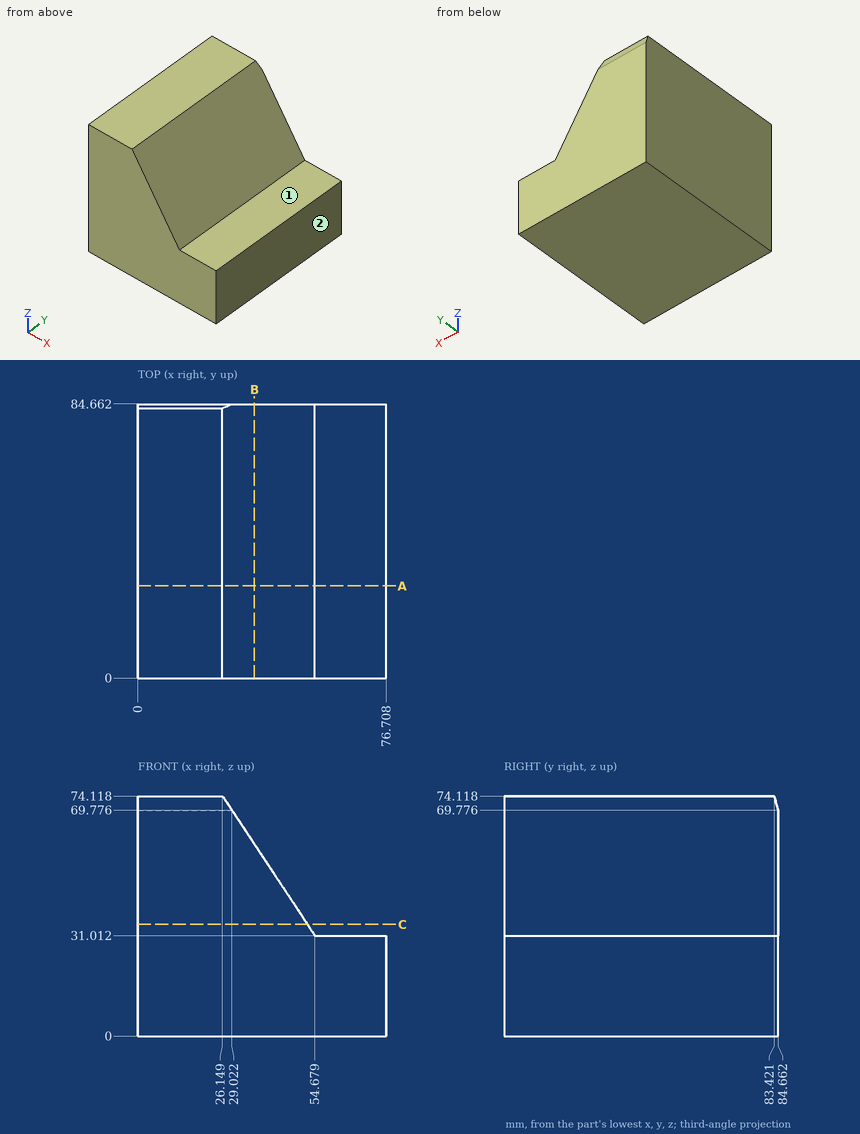
Verification items for this drawing (mm, ordinates from the low corner). A direction names the side the tool comes from. Give positions to 0.01 mm unless a question says otherwise; leave off trailing zeros. Write each loop counter-clockwise with the first axis right and the second up, starting at its lowest first coordinate (ties: lowest second). Pieces come first, ordered by that corner, then holes.
1) Thickness scan on line 1 (Z direction, x = 58, y = 28.5); line 2 (X direction, y = 72, z = 67.5); line 3 (X direction, y = 36.5, z = 61.5). Record the ranges inside material, lowest first.
Values follow:
line 1: z = 0 to 31.01
line 2: x = 0 to 30.53
line 3: x = 0 to 34.5
2) Cross-section at A-A (y = 28.5). Record the boundary of the cut face in (x, z), plus the area to 3 significant figures.
Values follow:
outline: (0, 0) - (76.71, 0) - (76.71, 31.01) - (54.68, 31.01) - (26.15, 74.12) - (0, 74.12) - close
area: 4,120 mm2
3) Cross-section at C-C (z = 34.5). Record the boundary of the cut face in (x, y).
Values follow:
outline: (0, 0) - (52.37, 0) - (52.37, 84.66) - (0, 84.66) - close
4) Go/stop test with flat-tipped pins: pin 1 Ø5 at (x, y) = (37, 70.5) entering from +Z; pin 2 Ø17.5 at (x, y) = (69.5, 58.5) entering from +Z; pin 3 Ø8 at (x, y) = (31, 49.5) entering from +Z. Record where each tip stops, or that it passes through.
Values follow:
pin 1: stops at z = 61.5
pin 2: stops at z = 31.01
pin 3: stops at z = 72.83
5) Cross-section at B-B (x = 36). Record the boundary of the cut face in (y, z).
Values follow:
outline: (0, 0) - (84.66, 0) - (84.66, 59.23) - (0, 59.23) - close
6) Set-up check for the marked faces 1 and 2: record each of +Z, -Z, +X, -X, +Y, -Y from which the full face is reachable in a straight line by a thin tool's end or side.
Values follow:
face 1: +Z, +X, +Y, -Y
face 2: +Z, -Z, +X, +Y, -Y
